Autodesk Inventor part; units mm, degrees
ref_plane "YZ Plane" through (0, 0, 0) normal (1, 0, 0) x (0, 1, 0)
ref_plane "XZ Plane" through (0, 0, 0) normal (0, 1, 0) x (-1, 0, 0)
ref_plane "XY Plane" through (0, 0, 0) normal (0, 0, 1) x (1, 0, 0)
sketch "Эскиз1" plane through (0, 0, 0) normal (1, 0, 0) x (0, 1, 0)
  circle A0 centre (0, 0) radius 132.5
  dimension "d0" = 265
extrude "Выдавливание1" add sketch "Эскиз1" along normal mid plane 31
sketch "Эскиз2" plane through (15.5, 0, 0) normal (1, 0, 0) x (0, 0, -1)
  circle A0 centre (0, 0) radius 76.5
  dimension "d3" = 153
extrude "Выдавливание2" add sketch "Эскиз2" along normal blind 62
sketch "Эскиз3" plane through (-15.5, 0, 0) normal (-1, 0, 0) x (0, 0, 1)
  circle A0 centre (0, 0) radius 76.5
  dimension "d6" = 153
extrude "Выдавливание3" add sketch "Эскиз3" along normal blind 62
sketch "Эскиз4" plane through (-77.5, 0, 0) normal (-1, 0, 0) x (0, 0, 1)
  circle A0 centre (0, 0) radius 45
  dimension "d9" = 90
extrude "Выдавливание4" cut sketch "Эскиз4" against normal through all
sketch "Эскиз5" plane through (0, 0, 0) normal (0, 0, 1) x (1, 0, 0)
  circle A0 centre (49.5, 0) radius 18.5
  line L0 (77.5, 45) -> (77.5, -45)
  point P0 (0, 0)
  dimension "d12" = 28
  dimension "d13" = 37
extrude "Выдавливание5" cut sketch "Эскиз5" along normal through all both and the other way through all
sketch "Эскиз7" plane through (15.5, 0, 0) normal (1, 0, 0) x (0, 0, -1)
  circle A0 centre (-109, 0) radius 11
  circle A1 centre (109, 0) radius 11
  point P0 (0, 0)
  dimension "d16" = 109
  dimension "d17" = 109
  dimension "d18" = 22
  dimension "d19" = 22
extrude "Выдавливание6" cut sketch "Эскиз7" against normal through all
sketch "Эскиз8" plane through (0, 0, 0) normal (0, 1, 0) x (-1, 0, 0)
  point P0 (0, 0)
properties part number "Переходник Чугун СЧ15"
Could you check a few things on this model? Use its own coordinates, in mm. A direction names the side the tool comes from. Give positions to 0.01 mm unless a question says otherwise; leave off trailing zeros. Order: outer loops, then holes, each group sorted by start corner. A loop starts at its lowest first (then second) coordinate and runs counter-clockwise, first axis right, second up. Notation, with made-up numbers: (74, 16.5) -> (115, 16.5) arc R16 cw to (115, 34.5) -> close; hole circle Ø5 at (-16, 4.25). An arc over 180 degrees is marked (long way). Return JSON: item names as keys, results as strings.
1. Imagine slicing it at D-D on x = -3. List the corners of the cut face in (y, z) for me.
Answer list:
{"outline": "circle Ø265 at (0, 0); hole circle Ø90 at (0, 0); hole circle Ø22 at (0, -109); hole circle Ø22 at (0, 109)"}
2. Imagine slicing it at A-A on y = 0. Give the number of separate pieces and of enclosed holes in the cut face, then the cut area to 3 significant figures.
Answer list:
{"separate pieces": "6", "enclosed holes": "0", "area": "9,540 mm2"}
3. Imagine slicing it at C-C on x = 55.5. List the corners of the cut face in (y, z) for me.
Answer list:
{"outline": "(-17.5, -74.47) -> (-17.5, -41.46) arc R45 cw to (-17.5, 41.46) -> (-17.5, 74.47) arc R76.5 ccw to start; (17.5, -74.47) arc R76.5 ccw to (17.5, 74.47) -> (17.5, 41.46) arc R45 cw to (17.5, -41.46) -> close"}
4. Thinking about a two-plate mould opening in Z: for faces 4 (the cylindrical face through (0, 0, -98)), 5 (the cylindrical face through (-46.066, 46.549, -60.708)), 6 (the flat face through (15.5, 57, -57)), which applies, pulls with the +Z half, pulls with the -Z half, needs draft (parallel to the pull), parting line crosses it, or undercut?
Answer list:
{"face 4": "undercut", "face 5": "parting line crosses it", "face 6": "needs draft"}
5. For pin 1 Ø12 at (x, z) = (-54.5, 7.5) entering from -Y; pin 2 Ø3 at (x, y) = (5, -45.5) entering from +Z; pin 3 Ø20 at (y, z) = (0, 109) entering from -X; pin 4 Ø1 at (x, y) = (47.5, 45.5) entering from +Z, each with a flat end and sliding along its axis, tell me the tip position at first contact or that it passes through.
Answer list:
{"pin 1": "stops at y = -76.49", "pin 2": "stops at z = 124.98", "pin 3": "passes through", "pin 4": "stops at z = 61.86"}
6. Imagine slicing it at B-B on z = 0. List the corners of the cut face in (x, y) for me.
Answer list:
{"outline": "(-77.5, -76.5) -> (-15.5, -76.5) -> (-15.5, -132.5) -> (15.5, -132.5) -> (15.5, -76.5) -> (77.5, -76.5) -> (77.5, -45) -> (-77.5, -45) -> close; (-77.5, 45) -> (77.5, 45) -> (77.5, 76.5) -> (15.5, 76.5) -> (15.5, 132.5) -> (-15.5, 132.5) -> (-15.5, 76.5) -> (-77.5, 76.5) -> close"}
7. I need wall thicknesses on line 1 (X direction, y = -93, z = 0.5); line 2 (Y direction, x = 40.5, z = 0); line 3 (Y direction, x = -48, z = -36). Which ranges of each line are inside material? Lowest first, please. Write a range as from..to.
Answer list:
{"line 1": "x = -15.5..15.5", "line 2": "y = -76.5..-45, 45..76.5", "line 3": "y = -67.5..-27, 27..67.5"}
8. On a 3-axis mill with a long thin cutter (end or side, diameter ignored), from which of +Z, -Z, +X, -X, +Y, -Y can I reach the whole of each face in a straight line? I mean faces 1 (the cylindrical face through (-1.085, -17.235, 41.569)), 2 (the flat face through (-15.5, 57, -57)), 3 (the cylindrical face through (46.066, -22.979, -72.967)). Say none if no direction works.
Answer list:
{"face 1": "+X, -X", "face 2": "-X", "face 3": "+X"}
